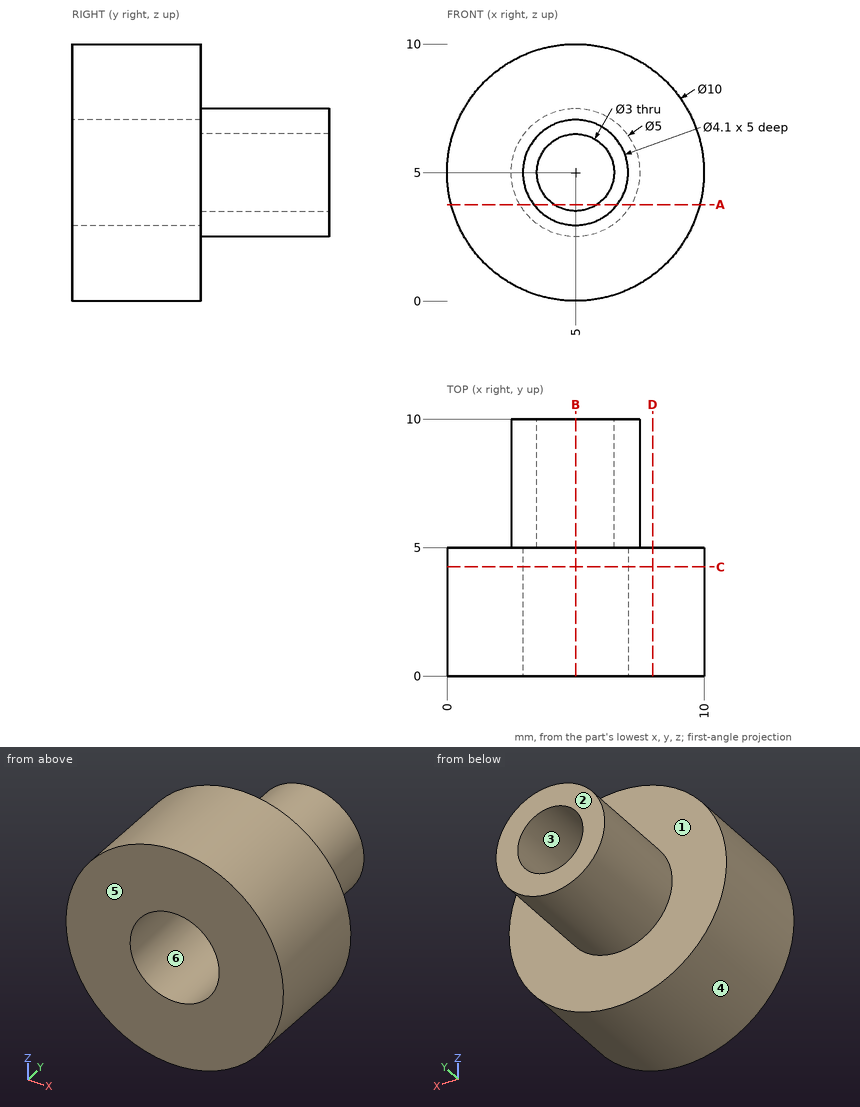
The drawing under review shows one solid part. Ordinate dimensions are in mm from its lowest x, y, z. A direction names the side the tool comes from. Coordinates: 2 decimals unless noted, no trailing zeros. Loops run counter-clockwise (first coordinate to the right, second up) from the corner with the lowest first, then second, coordinate; pieces in that order, holes last. Notation, with made-up numbers: (-10, 43.5) - (6, 43.5) arc R25 ccw to (6, 56.5) - close; hole circle Ø4 at (74, -14). An arc over 180 degrees is marked (long way). Return JSON: item names as keys, results as strings.
Item 1: For the marked faces 1 and 2, list the 3-axis set-ups (+Z, -Z, +X, -X, +Y, -Y) from which the entire face can be reached by the end or side of a thin tool; tool diameter is ignored.
Determined:
{"face 1": "+Y", "face 2": "+Z, -Z, +X, -X, +Y"}
Item 2: Take a section at D-D (x = 8). Give the boundary of the cut face in (y, z), then the cut area to 3 significant figures.
Determined:
{"outline": "(0, 1) - (5, 1) - (5, 9) - (0, 9) - close", "area": "40.0 mm2"}
Item 3: For line 1 (Y direction, x = 6.75, z = 9.25); line 2 (X direction, y = 8.5, z = 5); line 3 (Z direction, x = 4.5, y = 8.5), list the stretches that pass through material, from the lowest coordinate up.
Determined:
{"line 1": "y = 0 to 5", "line 2": "x = 2.5 to 3.5, 6.5 to 7.5", "line 3": "z = 2.55 to 3.59, 6.41 to 7.45"}
Item 4: Take a section at B-B (x = 5). Give the boundary of the cut face in (y, z).
Determined:
{"outline": "(0, 0) - (5, 0) - (5, 2.5) - (10, 2.5) - (10, 3.5) - (5, 3.5) - (5, 2.95) - (0, 2.95) - close; (0, 7.05) - (5, 7.05) - (5, 6.5) - (10, 6.5) - (10, 7.5) - (5, 7.5) - (5, 10) - (0, 10) - close"}
Item 5: Insertion check: pin 1 (3.5 mm diameter, centred on x = 5, z = 5, fed in from -Y); pin 2 (5.5 mm diameter, centred on x = 5, z = 5, fed in from -Y); pin 3 (1 mm diameter, centred on y = 2.5, z = 3, fed in from -X). Each pin has a flat end and moves straight along its axis. Give the tip position at first contact, or say it passes through.
Determined:
{"pin 1": "stops at y = 5", "pin 2": "stops at y = 0", "pin 3": "stops at x = 0.23"}
Item 6: Mouldability with a two-part tool opening along Z and no side actions: class the marked faces 3, 4, 5 and 6 as pulls with the +Z half, pulls with the -Z half, needs draft (parallel to the pull), parting line crosses it, or undercut.
Determined:
{"face 3": "undercut", "face 4": "parting line crosses it", "face 5": "needs draft", "face 6": "undercut"}
Item 7: Take a section at C-C (y = 4.25). Give the boundary of the cut face in (x, z).
Determined:
{"outline": "circle Ø10 at (5, 5); hole circle Ø4.1 at (5, 5)"}
Item 8: Take a section at A-A (z = 3.75). Give the boundary of the cut face in (x, y).
Determined:
{"outline": "(0.16, 0) - (3.38, 0) - (3.38, 5) - (4.17, 5) - (4.17, 10) - (2.83, 10) - (2.83, 5) - (0.16, 5) - close; (5.83, 5) - (6.62, 5) - (6.62, 0) - (9.84, 0) - (9.84, 5) - (7.17, 5) - (7.17, 10) - (5.83, 10) - close"}
